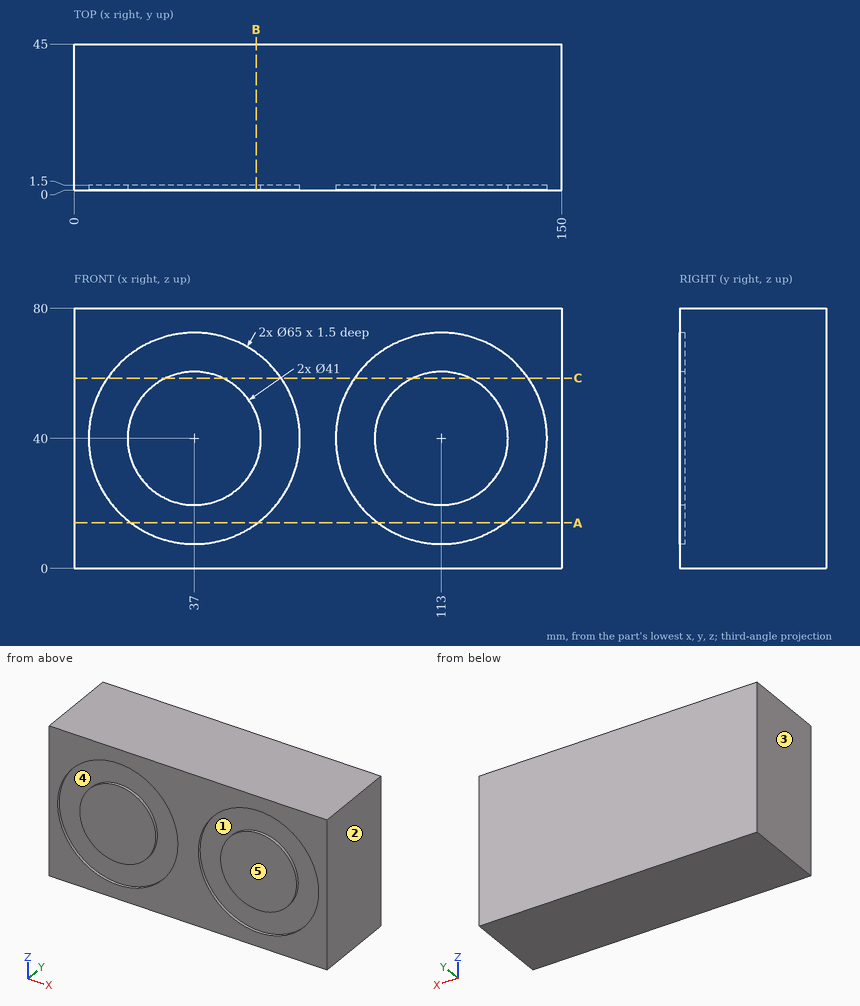
Part print with two shaded views. Sizes in mm from the minimum x, y, z corner. A direction names the side the tool comes from. Give positions to 0.01 mm unless a question says otherwise; leave off trailing zeros. Order: outer loops, then holes, each group sorted by start corner. A loop starts at its lowest first (then second) coordinate and runs counter-clockwise, first axis right, second up.
1) Mould opens along X. For the marked faces 1, 2 and 3 say: +X half, -X half, draft (parallel to the pull), parting line (faces both ways), or undercut.
2) Saw through at C-C, the plane z = 58.5. Write the cut outline in (x, y).
3) Wall check: probe 1 along Z at (x, y) = (37, 0.5); probe 2 along Y at (x, z) = (20, 52). Give the ranges that are in metal, low to high.
4) 3-axis set-ups, long thin cutter, end or side, ignore diameter. For the marked faces 4 and 5: which of +Z, -Z, +X, -X, +Y, -Y reach the whole face in a straight line?
5) Saw through at B-B, the plane x = 56. Write the cut outline in (y, z).
6) Saw through at A-A, the plane z = 14. Write the cut outline in (x, y), then the cut area to 3 significant figures.
Computed:
1. face 1: undercut
1. face 2: +X half
1. face 3: -X half
2. outline: (0, 0) - (10.28, 0) - (10.28, 1.5) - (28.17, 1.5) - (28.17, 0) - (45.83, 0) - (45.83, 1.5) - (63.72, 1.5) - (63.72, 0) - (86.28, 0) - (86.28, 1.5) - (104.17, 1.5) - (104.17, 0) - (121.83, 0) - (121.83, 1.5) - (139.72, 1.5) - (139.72, 0) - (150, 0) - (150, 45) - (0, 45) - close
3. probe 1: z = 0 to 7.5, 19.5 to 60.5, 72.5 to 80
3. probe 2: y = 1.5 to 45
4. face 4: -Y
4. face 5: +Z, -Z, +X, -X, -Y
5. outline: (0, 0) - (45, 0) - (45, 80) - (0, 80) - (0, 66.37) - (1.5, 66.37) - (1.5, 47.7) - (0, 47.7) - (0, 32.3) - (1.5, 32.3) - (1.5, 13.63) - (0, 13.63) - close
6. outline: (0, 0) - (17.5, 0) - (17.5, 1.5) - (56.5, 1.5) - (56.5, 0) - (93.5, 0) - (93.5, 1.5) - (132.5, 1.5) - (132.5, 0) - (150, 0) - (150, 45) - (0, 45) - close
6. area: 6,630 mm2
